```python
from build123d import *

# Parameters (mm, degrees)
F1_DEPTH      = 25.4
F2_START      = -381
F2_DEPTH      = 25.4
F3_W          = 12.7
F3_H          = 38.1
F4_DEPTH      = 361.95
F4_DEPTH_BACK = 6.35
F6_DEPTH      = 6.35
F7_START      = -400.05
F7_DEPTH      = 6.35


# Not quite as in the source:
# - a feature of the source that left no trace in its solid (it failed there, or was rolled back) is left out


with BuildPart() as f1:
    # F0 (on Front) → F1 (new body)
    with BuildSketch(Plane.XZ):
        with BuildLine():
            Line((-11.43, 174.7373407305), (-11.43, 0))
            ThreePointArc((-11.43, 0), (0, -11.43), (11.43, 0))
            Line((11.43, 0), (11.43, 231.14))
            ThreePointArc((11.43, 231.14), (5.715, 241.0386703653), (-5.715, 241.0386703653))
            Line((-5.715, 241.0386703653), (-38.7105678842, 221.9886703653))
            Line((-38.7105678842, 221.9886703653), (-11.43, 174.7373407305))
        make_face()
        with BuildLine():
            Line((-3.571875, 0), (-3.571875, 231.14))
            ThreePointArc((-3.571875, 231.14), (0, 234.711875), (3.571875, 231.14))
            Line((3.571875, 231.14), (3.571875, 0))
            ThreePointArc((3.571875, 0), (0, -3.571875), (-3.571875, 0))
        make_face(mode=Mode.SUBTRACT)
        with BuildLine():
            ThreePointArc((3.571875, 231.14), (0, 234.711875), (-3.571875, 231.14))
            Line((-3.571875, 231.14), (-3.571875, 0))
            ThreePointArc((-3.571875, 0), (0, -3.571875), (3.571875, 0))
            Line((3.571875, 0), (3.571875, 231.14))
        make_face()
    extrude(amount=-F1_DEPTH)



with BuildPart() as f2:
    # F0 (on Front) → F2 (new body)
    with BuildSketch(Plane.XZ.offset(F2_START)):
        with BuildLine():
            Line((-11.43, 174.7373407305), (-11.43, 0))
            ThreePointArc((-11.43, 0), (0, -11.43), (11.43, 0))
            Line((11.43, 0), (11.43, 231.14))
            ThreePointArc((11.43, 231.14), (5.715, 241.0386703653), (-5.715, 241.0386703653))
            Line((-5.715, 241.0386703653), (-38.7105678842, 221.9886703653))
            Line((-38.7105678842, 221.9886703653), (-11.43, 174.7373407305))
        make_face()
        with BuildLine():
            Line((-3.571875, 0), (-3.571875, 231.14))
            ThreePointArc((-3.571875, 231.14), (0, 234.711875), (3.571875, 231.14))
            Line((3.571875, 231.14), (3.571875, 0))
            ThreePointArc((3.571875, 0), (0, -3.571875), (-3.571875, 0))
        make_face(mode=Mode.SUBTRACT)
        with BuildLine():
            ThreePointArc((3.571875, 231.14), (0, 234.711875), (-3.571875, 231.14))
            Line((-3.571875, 231.14), (-3.571875, 0))
            ThreePointArc((-3.571875, 0), (0, -3.571875), (3.571875, 0))
            Line((3.571875, 0), (3.571875, 231.14))
        make_face()
    extrude(amount=-F2_DEPTH)


with BuildPart() as f1_1:
    add(f1.part)

    add(f2.part)  # F4 merges F2
    # F3 (on face) → F4 (join, two sides)
    with BuildSketch(Plane(origin=(0, 25.4, 0), x_dir=(-1, 0, 0), z_dir=(0, 1, 0))) as f4_sk:
        with Locations((0, 155.6873407305)):
            Rectangle(F3_W, F3_H)
        with Locations((0, 19.05)):
            Rectangle(F3_W, F3_H)
    extrude(amount=F4_DEPTH)
    extrude(f4_sk.sketch, amount=-F4_DEPTH_BACK)

    # F0 (on Front) → F6 (cut)
    with BuildSketch(Plane.XZ):
        with BuildLine():
            ThreePointArc((3.571875, 231.14), (0, 234.711875), (-3.571875, 231.14))
            Line((-3.571875, 231.14), (-3.571875, 0))
            ThreePointArc((-3.571875, 0), (0, -3.571875), (3.571875, 0))
            Line((3.571875, 0), (3.571875, 231.14))
        make_face()
    extrude(amount=-F6_DEPTH, mode=Mode.SUBTRACT)

    # F0 (on Front) → F7 (cut)
    with BuildSketch(Plane.XZ.offset(F7_START)):
        with BuildLine():
            ThreePointArc((3.571875, 231.14), (0, 234.711875), (-3.571875, 231.14))
            Line((-3.571875, 231.14), (-3.571875, 0))
            ThreePointArc((-3.571875, 0), (0, -3.571875), (3.571875, 0))
            Line((3.571875, 0), (3.571875, 231.14))
        make_face()
    extrude(amount=-F7_DEPTH, mode=Mode.SUBTRACT)


solid = f1_1.part
```
Can you work these out from the model? Positions are in its coordinate system, mm. A direction names the side the tool comes from. Coordinates: 2 decimals unless noted, no trailing zeros. Loops run counter-clockwise (first coordinate to the right, second up) from the corner with the lowest first, then second, coordinate; pieces in that order, holes last. Notation, with made-up numbers: (41, 58) -> (81, 58) arc R18 cw to (81, 72) -> close; hole circle Ø4 at (-39.5, 31). An arc over 180 degrees is marked (long way). Answer as a JSON object with one key per item and string values.
1) Imagine slicing it at C-C (x = -16). Please give me the cut outline in (y, z), then the cut area to 3 significant figures.
Results:
{"outline": "(0, 182.65) -> (25.4, 182.65) -> (25.4, 235.1) -> (0, 235.1) -> close; (381, 182.65) -> (406.4, 182.65) -> (406.4, 235.1) -> (381, 235.1) -> close", "area": "2,660 mm^2"}
2) Imagine slicing it at A-A (y = 311.5). Please give me the cut outline in (x, z), then the cut area to 3 significant figures.
Results:
{"outline": "(-6.35, 0) -> (6.35, 0) -> (6.35, 38.1) -> (-6.35, 38.1) -> close; (-6.35, 136.64) -> (6.35, 136.64) -> (6.35, 174.74) -> (-6.35, 174.74) -> close", "area": "968 mm^2"}
3) Imagine slicing it at D-D (z = 208.5). Please give me the cut outline in (x, y).
Results:
{"outline": "(-30.92, 0) -> (-3.57, 0) -> (-3.57, 6.35) -> (3.57, 6.35) -> (3.57, 0) -> (11.43, 0) -> (11.43, 25.4) -> (-30.92, 25.4) -> close; (-30.92, 381) -> (11.43, 381) -> (11.43, 406.4) -> (3.57, 406.4) -> (3.57, 400.05) -> (-3.57, 400.05) -> (-3.57, 406.4) -> (-30.92, 406.4) -> close"}
4) If I drill on line 1 (Z direction, x = -3.5, y = 121); line 2 (Y direction, x = 1, z = 182); line 3 (Y direction, x = -7, z = 229), over which ranges is the centre line in solid material (lowest first)?
Results:
{"line 1": "z = 0 to 38.1, 136.64 to 174.74", "line 2": "y = 6.35 to 25.4, 381 to 400.05", "line 3": "y = 0 to 25.4, 381 to 406.4"}
5) Imagine slicing it at B-B (z = 132). Please give me the cut outline in (x, y), then the cut area to 3 significant figures.
Results:
{"outline": "(-11.43, 0) -> (-3.57, 0) -> (-3.57, 6.35) -> (3.57, 6.35) -> (3.57, 0) -> (11.43, 0) -> (11.43, 25.4) -> (-11.43, 25.4) -> close; (-11.43, 381) -> (11.43, 381) -> (11.43, 406.4) -> (3.57, 406.4) -> (3.57, 400.05) -> (-3.57, 400.05) -> (-3.57, 406.4) -> (-11.43, 406.4) -> close", "area": "1,070 mm^2"}
6) For faces 5 (the face through (-11.43, 394, 89)), 6 (the face through (0, 201, 0)), 7 (the face through (0, 201, 136.637)), 8 (the face through (6.35, 201, 155)), which set-ups out of +Z, -Z, +X, -X, +Y, -Y let a thin tool reach every point of the face, with its end or its side?
Results:
{"face 5": "-Z, -X, +Y, -Y", "face 6": "-Z, +X, -X", "face 7": "+X, -X", "face 8": "+Z, -Z, +X"}
7) For P1, Ø20.5, axis at y = 14.5, z = 119.5, coming from the -X side; P2, Ø6.5, axis at x = -1.5, y = 133.5, coming from the +Z side; P3, Ø25, axis at x = -25, z = 83.5, coming from the +Y side; P4, Ø8, axis at y = 287, z = 175.5, coming from the -X side, each with a flat end and sliding along its axis, tell me the tip position at first contact or that it passes through.
Results:
{"P1": "stops at x = -11.43", "P2": "stops at z = 174.74", "P3": "passes through", "P4": "stops at x = -6.35"}
8) Thinking about a two-plate mould opening in Z: for faces 1 (the face through (-8, 25.4, 146)), 2 (the face through (-0.251, 12.522, -11.427)), 3 (the face through (-6.35, 201, 19)), 4 (the face through (-21.98, 12.52, 231.65)), which applies, pulls with the +Z half, pulls with the -Z half, needs draft (parallel to the pull), parting line crosses it, or undercut?
Results:
{"face 1": "undercut", "face 2": "pulls with the -Z half", "face 3": "needs draft", "face 4": "pulls with the +Z half"}
